Could you check a few things on this drawing? It's one solid part, dimensions in mm from its lowest x, y, z. A direction names the side the tool comes from. Coordinates: 2 decimals unless noted, no trailing zeros. Loops run counter-clockwise (first coordinate to the right, second up) from the corner with the lowest first, then second, coordinate; pieces in that order, holes last. Notation, with made-up numbers: M 31,-35.5 L 67,-35.5 A26 ccw 67,1.5 Z; hole C -4,10.25 d11. An arc over 180 degrees is marked long. Use one line per item in the form item = value. Start each with the question number.
(1) Thinking about a two-plate mould opening in Y: for the marked faces 3, 4, 5 and 6, which applies, +Y half, -Y half, draft (parallel to the pull), parting line (faces both ways), or undercut?
(2) Imagine slicing it at D-D, the plane y = 25. Please give me the cut outline in (x, z), and give its area (3 significant figures).
(3) Will these pins go through, and if not, where does the flat tip stop? P1, Ø3, axis at y = 18.5, z = 20.5, coming from the -X side; P2, Ø5, axis at x = 32, y = 43, coming from the +Z side; P3, Ø13, axis at x = 40, y = 36, coming from the -Z side.
(4) On a 3-axis mill with a long thin cutter (end or side, diameter ignored), from which of +Z, -Z, +X, -X, +Y, -Y can I reach the whole of each face in a straight line? I mean the marked faces 1 and 2. Say none if no direction works.
(5) Imagine slicing it at A-A, the plane x = 27. Please give me the cut outline in (y, z).
(6) Please list where these lines run through material, in increasing order: L1, parallel to X at y = 40, z = 19.5; L2, parallel to Y at x = 48, z = 5; L3, parallel to Z at x = 68.5, y = 6.
(7) Imagine slicing it at C-C, the plane z = 18.25. Please give me the cut outline in (x, y), and give its area (3 significant figures).
(8) Imagine slicing it at B-B, the plane y = 5. Please give me the cut outline in (x, z), and give its area (3 significant figures).
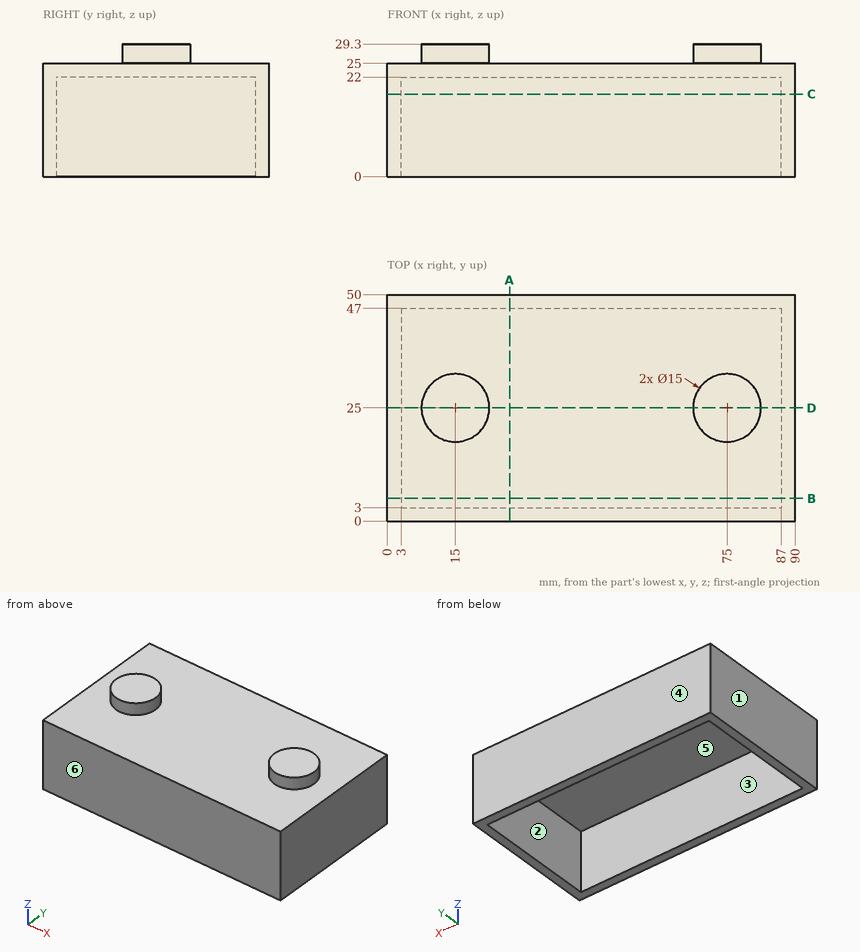
Answer:
q1.face_3 = undercut
q1.face_4 = +Y half
q1.face_5 = undercut
q1.face_6 = -Y half
q2.outline = M 0,0 L 3,0 L 3,22 L 87,22 L 87,0 L 90,0 L 90,25 L 82.5,25 L 82.5,29.3 L 67.5,29.3 L 67.5,25 L 22.5,25 L 22.5,29.3 L 7.5,29.3 L 7.5,25 L 0,25 Z
q2.area = 531 mm²
q3.P1 = 0
q3.P2 = 25
q3.P3 = 22
q4.face_1 = +Z, -Z, -X, +Y, -Y
q4.face_2 = -Z
q5.outline = M 0,0 L 3,0 L 3,22 L 47,22 L 47,0 L 50,0 L 50,25 L 0,25 Z
q6.L1 = 0 to 3, 87 to 90
q6.L2 = 0 to 3, 47 to 50
q6.L3 = 22 to 25
q7.outline = M 0,0 L 90,0 L 90,50 L 0,50 Z; hole M 3,3 L 87,3 L 87,47 L 3,47 Z
q7.area = 804 mm²
q8.outline = M 0,0 L 3,0 L 3,22 L 87,22 L 87,0 L 90,0 L 90,25 L 0,25 Z
q8.area = 402 mm²
